```python
from build123d import *

# Parameters (mm, degrees)
SKETCH1_R           = 17.5
BOSS_EXTRUDE1_DEPTH = 2.5
BOSS_EXTRUDE2_DEPTH = 8
SKETCH3_R           = 4
BOSS_EXTRUDE3_DEPTH = 24.5
BOSS_EXTRUDE4_START = 12
SKETCH7_R           = 4
BOSS_EXTRUDE4_DEPTH = 12
BOSS_EXTRUDE5_DEPTH = 20
SKETCH10_R          = 1.55
CUT_EXTRUDE1_DEPTH  = 6.1
SKETCH11_R          = 1.55
CUT_EXTRUDE4_DEPTH  = 6.1


with BuildPart() as part:
    # Sketch1 → Boss-Extrude1 (new, symmetric)
    with BuildSketch(Plane.XY):
        Circle(SKETCH1_R)
    extrude(amount=BOSS_EXTRUDE1_DEPTH, both=True)

    # Sketch2 → Boss-Extrude2 (add)
    with BuildSketch(Plane.XY.offset(2.5)):
        with BuildLine():
            Line((7.875, 13.63990011), (4.125, 7.144709581))
            ThreePointArc((4.125, 7.144709581), (0, 8.25), (-4.125, 7.144709581))
            Line((-4.125, 7.144709581), (-7.875, 13.63990011))
            ThreePointArc((-7.875, 13.63990011), (0, 15.75), (7.875, 13.63990011))
        make_face()
    extrude(amount=BOSS_EXTRUDE2_DEPTH)

    # Sketch3 → Boss-Extrude3 (add)
    with BuildSketch(Plane.XY.offset(2.5)):
        Circle(SKETCH3_R)
    extrude(amount=BOSS_EXTRUDE3_DEPTH)

    # Sketch7 → Boss-Extrude4 (add)
    with BuildSketch(Plane(origin=(0, 0, -2.5), x_dir=(-1, 0, 0), z_dir=(0, 0, -1)).offset(BOSS_EXTRUDE4_START)):
        with Locations(Location((0, 0, 0), (0, 0, 180))):
            Circle(SKETCH7_R)
    extrude(amount=-BOSS_EXTRUDE4_DEPTH)

    # Sketch9 → Boss-Extrude5 (add)
    with BuildSketch(Plane(origin=(0, 0, -14.5), x_dir=(-1, 0, 0), z_dir=(0, 0, -1))):
        Polygon((0, 3.5), (-3.031088913, 1.75), (-3.031088913, -1.75), (0, -3.5), (3.031088913, -1.75), (3.031088913, 1.75), align=None)
    extrude(amount=BOSS_EXTRUDE5_DEPTH)

    # Sketch10 → Cut-Extrude1 (cut)
    with BuildSketch(Plane(origin=(-1.515544457, -2.625, 0), x_dir=(0.866025403784435, -0.5000000000000062, 0), z_dir=(-0.5000000000000062, -0.866025403784435, 0))):
        with Locations((0, -29.5)):
            Circle(SKETCH10_R)
    extrude(amount=-CUT_EXTRUDE1_DEPTH, mode=Mode.SUBTRACT)

    # Sketch11 → Cut-Extrude4 (cut)
    with BuildSketch(Plane(origin=(1.515544457, -2.625, 0), x_dir=(0, 0, 1), z_dir=(-0.49999999999999717, 0.8660254037844404, 0))):
        with Locations(Location((-25.5, 0, 0), (0, 0, 90))):
            Circle(SKETCH11_R)
    extrude(amount=CUT_EXTRUDE4_DEPTH, mode=Mode.SUBTRACT)


solid = part.part
```
Check sheet for the modelled part. Datum: model origin and axes. Units: mm. A direction names the side the tool comes from. Give positions to 0.01 mm unless a question says otherwise; leave off trailing zeros. Order: outer loops, then holes, each group sorted by start corner. A loop starts at its lowest first (then second) coordinate and runs counter-clockwise, first axis right, second up. Notation, with made-up numbers: M 81.25,57 L 93.25,57 A11 ccw 93.25,77 Z; hole C 32.25,69.5 d3. An arc over 180 degrees is marked long. Answer in a Markdown table with one row per item.
1) Cross-section at A-A, the plane z = 8. Enter the section's corners in (x, y) (3 decimals), plus the area to 3 significant figures.
Filled sheet:
| item | result |
|---|---|
| outline | M -7.875,13.64 L -4.125,7.145 A8.25 cw 4.125,7.145 L 7.875,13.64 A15.75 ccw Z; C 0,0 d8 |
| area | 145 mm2 |
2) Cross-section at B-B, the plane y = 9.5. Enter the section's corners in (x, z), plus the area to 3 significant figures.
Filled sheet:
| item | result |
|---|---|
| outline | M -14.7,-2.5 L 14.7,-2.5 L 14.7,2.5 L 5.48,2.5 L 5.48,10.5 L -5.48,10.5 L -5.48,2.5 L -14.7,2.5 Z |
| area | 235 mm2 |
3) Gauge pin test, flat ends, axial feed: P1, Ø3, axis at y = -1, z = -27, coming from the +X side; P2, Ø4, axis at y = 7.5, z = 3.5, coming from the +X side; P3, Ø3, axis at x = -1.5, y = -7.5, coming from the -Z side. Record the tip position at first contact, or that the pin passes through.
Filled sheet:
| item | result |
|---|---|
| P1 | stops at x = 3.03 |
| P2 | stops at x = 16.52 |
| P3 | stops at z = -2.5 |
4) Access from +Z, -Z, +X, -X, +Y, -Y to the whole of each face (thin tool, end or side, straight path). Record for faces 4 (the flat face through (0.19, -3.39, -24.36)), 5 (the flat face through (-0.19, 3.39, -24.36)), 6 (the flat face through (-1.49, -2.64, -24.36)).
Filled sheet:
| item | result |
|---|---|
| face 4 | -Z, +X, -Y |
| face 5 | -Z, -X, +Y |
| face 6 | -Z, -X, -Y |
5) Thickness scan on L1, parallel to Y at x = 0, z = 16; L2, parallel to Z at x = 8, y = -6.5; L3, parallel to Z at x = 3, y = 2. Record the ranges inside material, lowest first. Write a range as [from, to].
Filled sheet:
| item | result |
|---|---|
| L1 | y = [-4, 4] |
| L2 | z = [-2.5, 2.5] |
| L3 | z = [-14.5, 27] |
6) Release check for a two-part mould opening along Z. For faces 1 (the flat face through (0, 0, -34.5)), 2 (the cylindrical face through (-0.867, 3.905, -8.584)), 3 (the cylindrical face through (-0.196, 0.064, -27.963)) record: +Z half, -Z half, draft (parallel to the pull), parting line (faces both ways), or undercut.
Filled sheet:
| item | result |
|---|---|
| face 1 | -Z half |
| face 2 | draft |
| face 3 | undercut |
7) Cross-section at C-C, the plane y = 0. Count the separate pieces of the cut face and the enclosed holes in it, plus the area to 3 significant figures.
Filled sheet:
| item | result |
|---|---|
| separate pieces | 1 |
| enclosed holes | 2 |
| area | 571 mm2 |
8) Cross-section at D-D, the plane z = 15. Enter the section's corners in (x, y), plus the area to 3 significant figures.
Filled sheet:
| item | result |
|---|---|
| outline | C 0,0 d8 |
| area | 50.3 mm2 |
